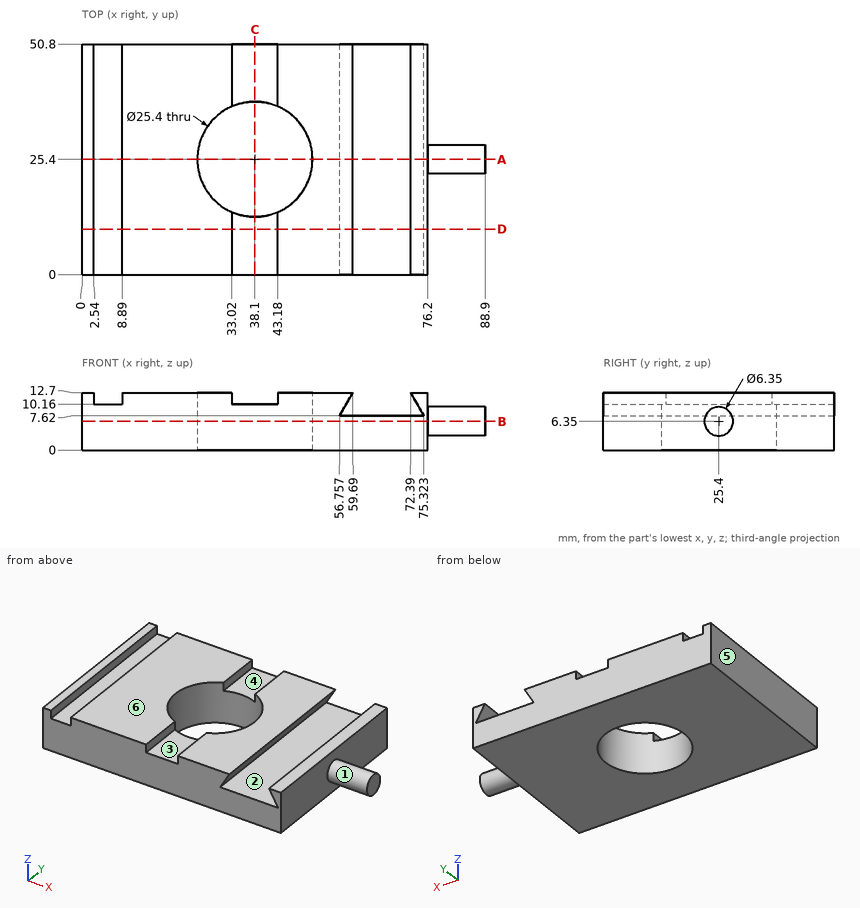
Geometry check sheet. Reference: drawing and pictorial views, mm from the part's lowest x, y, z. A direction names the side the tool comes from. Coordinates: 2 decimals unless noted, no trailing zeros. Order: outer loops, then holes, each group sorted by start corner. A loop starts at its lowest first (then second) coordinate and runs counter-clockwise, first axis right, second up. Notation, with made-up numbers: (17, 74.25) -> (68, 74.25) arc R15 ccw to (68, 80.25) -> close; hole circle Ø8 at (70.5, 21). An arc over 180 degrees is marked (long way). Write item = value, one per line. Start each with the question number.
1) Cross-section at B-B (z = 6.35). Enter the section's corners in (x, y) (3 decimals), then the cut area to 3 significant figures.
2) Go/stop test with a flat-tipped pin: P1, Ø2, axis at y = 5.5, z = 11.5, coming from the +X side. Record where the tip stops, or that it passes through.
3) Cross-section at C-C (x = 38.1). Enter the section's corners in (y, z), then the cut area to 3 significant figures.
4) Material ranges on L1, parallel to Y at x = 38.1, z = 5.25; L2, parallel to X at y = 25.4, z = 4.5; L3, parallel to X at y = 25.4, z = 3, recorded low to high.
5) Cross-section at A-A (y = 25.4). Enter the section's corners in (x, z) (3 decimals).
6) Mould release check, pull along X, two halves, no side actions. Record for the marked faces 4, 5 and 6: +X half, -X half, draft (parallel to the pull), parting line (faces both ways), or undercut.
7) Access from +Z, -Z, +X, -X, +Y, -Y to the whole of each face (thin tool, end or side, straight path). Record for the marked faces 1, 2 and 3.
8) Cross-section at D-D (y = 10). Enter the section's corners in (x, z).
Ans:
q1.outline = (0, 0) -> (76.2, 0) -> (76.2, 22.225) -> (88.9, 22.225) -> (88.9, 28.575) -> (76.2, 28.575) -> (76.2, 50.8) -> (0, 50.8) -> close; hole circle Ø25.4 at (38.1, 25.4)
q1.area = 3,440 mm²
q2.P1 = 76.2
q3.outline = (0, 0) -> (12.7, 0) -> (12.7, 10.16) -> (0, 10.16) -> close; (38.1, 0) -> (50.8, 0) -> (50.8, 10.16) -> (38.1, 10.16) -> close
q3.area = 258 mm²
q4.L1 = 0 to 12.7, 38.1 to 50.8
q4.L2 = 0 to 25.4, 50.8 to 88.9
q4.L3 = 0 to 25.4, 50.8 to 76.2
q5.outline = (0, 0) -> (25.4, 0) -> (25.4, 12.7) -> (8.89, 12.7) -> (8.89, 10.16) -> (2.54, 10.16) -> (2.54, 12.7) -> (0, 12.7) -> close; (50.8, 0) -> (76.2, 0) -> (76.2, 3.175) -> (88.9, 3.175) -> (88.9, 9.525) -> (76.2, 9.525) -> (76.2, 12.7) -> (72.39, 12.7) -> (75.323, 7.62) -> (56.757, 7.62) -> (59.69, 12.7) -> (50.8, 12.7) -> close
q6.face_4 = undercut
q6.face_5 = -X half
q6.face_6 = draft
q7.face_1 = +X
q7.face_2 = +Y, -Y
q7.face_3 = +Z, +Y, -Y
q8.outline = (0, 0) -> (76.2, 0) -> (76.2, 12.7) -> (72.39, 12.7) -> (75.32, 7.62) -> (56.76, 7.62) -> (59.69, 12.7) -> (43.18, 12.7) -> (43.18, 10.16) -> (33.02, 10.16) -> (33.02, 12.7) -> (8.89, 12.7) -> (8.89, 10.16) -> (2.54, 10.16) -> (2.54, 12.7) -> (0, 12.7) -> close
